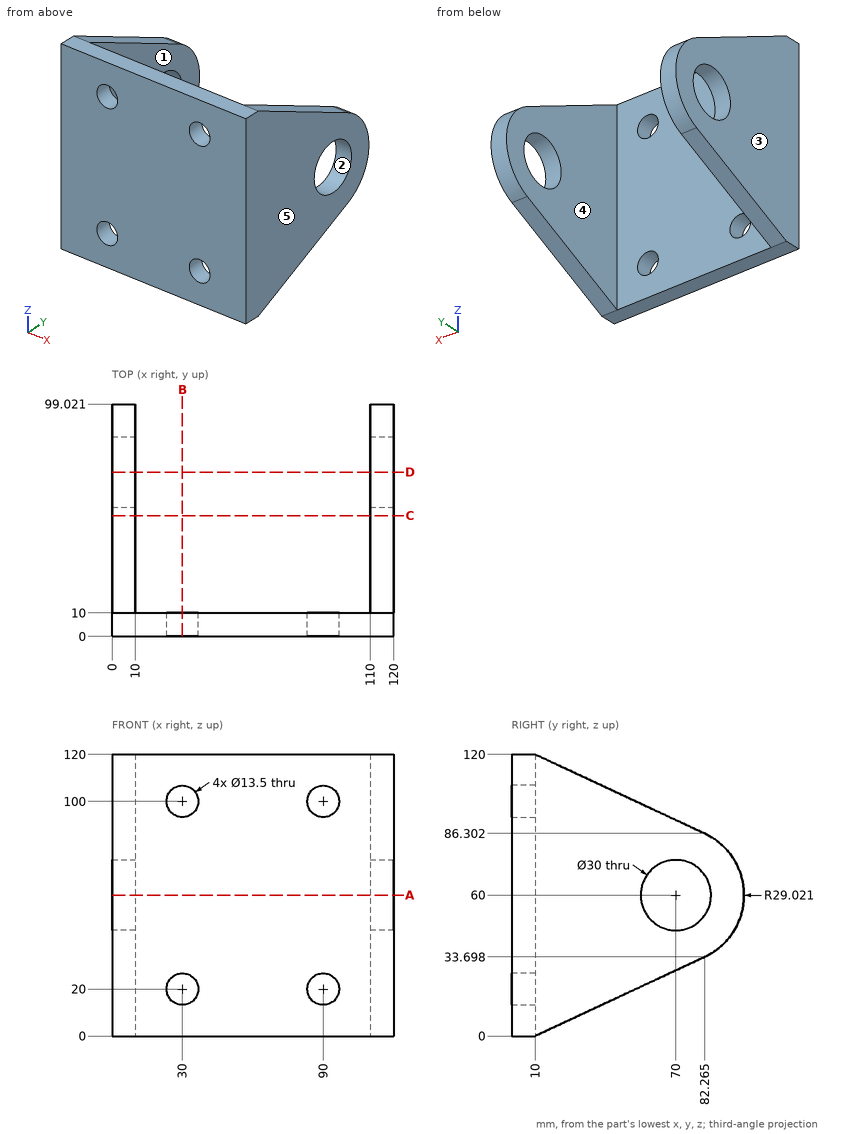
Source: three-view drawing plus pictorial views. Frame: mm from the lowest corner of the part. A direction names the side the tool comes from. Give positions to 0.01 mm unless a question says otherwise; leave off trailing zeros. Loops run counter-clockwise (first coordinate to the right, second up) from the corner with the lowest first, then second, coordinate; pieces in that order, holes last. Notation, with made-up numbers: M 40.5,73.25 L 49.5,73.25 A18 cw 49.5,94.25 Z; hole C 9,65.5 d8. An arc over 180 degrees is marked long. Use CSV: the item, a comma, the result in double quotes.
(1) Section B-B, the plane x = 30. Return loops of the section in (y, z), plus the area to 3 significant figures.
Outcome:
outline,"M 0,0 L 10,0 L 10,13.25 L 0,13.25 Z; M 0,26.75 L 10,26.75 L 10,93.25 L 0,93.25 Z; M 0,106.75 L 10,106.75 L 10,120 L 0,120 Z"
area,"930 mm²"
(2) Section A-A, the plane z = 60. Return loops of the section in (x, y).
Outcome:
outline,"M 0,0 L 120,0 L 120,55 L 110,55 L 110,10 L 10,10 L 10,55 L 0,55 Z; M 0,85 L 10,85 L 10,99.02 L 0,99.02 Z; M 110,85 L 120,85 L 120,99.02 L 110,99.02 Z"
(3) Pin query (flat end, axial travel): P1, Ø5, axis at x = 45.5, z = 33, coming from the +Y side. Return the tip coordinate at first contact, or that it passes through.
Outcome:
P1,"stops at y = 10"
(4) Section D-D, the plane y = 70. Return loops of the section in (x, z), plus the area to 3 significant figures.
Outcome:
outline,"M 0,27.98 L 10,27.98 L 10,45 L 0,45 Z; M 0,75 L 10,75 L 10,92.02 L 0,92.02 Z; M 110,27.98 L 120,27.98 L 120,45 L 110,45 Z; M 110,75 L 120,75 L 120,92.02 L 110,92.02 Z"
area,"681 mm²"
(5) Pull-direction query (X, two-part tool) for the marked faces 1, 2 and 3; classes: pulls with the +X half, pulls with the -X half, needs draft (parallel to the pull), parting line crosses it, or undercut.
Outcome:
face 1,"undercut"
face 2,"needs draft"
face 3,"pulls with the -X half"
(6) Set-up query: the marked faces 4 and 5. Return all of +Z, -Z, +X, -X, +Y, -Y with unobstructed straight access to the full face (end or side cutting, diameter ignored); none if empty.
Outcome:
face 4,"+Z, -Z, +Y"
face 5,"+Z, -Z, +X, +Y, -Y"
(7) Section C-C, the plane y = 51.5. Return loops of the section in (x, z).
Outcome:
outline,"M 0,19.35 L 10,19.35 L 10,100.65 L 0,100.65 Z; M 110,19.35 L 120,19.35 L 120,100.65 L 110,100.65 Z"
(8) Material intervals for L1, parallel to X at y = 2.5, z = 100; L2, parallel to Y at x = 7, z = 60; L3, parallel to X at y = 19, z = 34, sorted ascending. Write a range as [from, to].
Outcome:
L1,"x = [0, 23.25], [36.75, 83.25], [96.75, 120]"
L2,"y = [0, 55], [85, 99.02]"
L3,"x = [0, 10], [110, 120]"
